from build123d import *

# Parameters (mm, degrees)
F1_DEPTH  = 31.6
F2_START  = 27.6
F2_DEPTH  = 4
F0_R      = 3.05
F3_DEPTH  = 2
F4_W      = 2.5
F4_H      = 19.6
F5_DEPTH  = 2
F7_DEPTH  = 3
F8_R      = 0.5
F9_DEPTH  = 25
F10_R     = 1.75
F11_DEPTH = 3
F13_DEPTH = 10
F15_DEPTH = 4


# Not quite as in the source:
# - a feature names something its author has since deleted; it is built from what else it names


with BuildPart() as f1:
    # F0 (on Top) → F1 (new body)
    with BuildSketch(Plane.XY):
        Polygon((31.25, -9), (31.25, 0), (29.25, 0), (29.25, -7), (-29.25, -7), (-29.25, 0), (-31.25, 0), (-31.25, -9), align=None)
        Polygon((31.25, 0), (31.25, 9), (-31.25, 9), (-31.25, 0), (-29.25, 0), (-29.25, 7), (29.25, 7), (29.25, 0), align=None)
    extrude(amount=F1_DEPTH)

    # F0 (on Top) → F2 (join)
    with BuildSketch(Plane.XY.offset(F2_START)):
        with BuildLine():
            Line((29, 0), (29.25, 0))
            Line((29.25, 0), (29.25, 7))
            Line((29.25, 7), (-29.25, 7))
            Line((-29.25, 7), (-29.25, 0))
            Line((-29.25, 0), (-29, 0))
            ThreePointArc((-29, 0), (-24.5, 4.5), (-20, 0))
            Line((-20, 0), (-16.1, 0))
            ThreePointArc((-16.1, 0), (-13.5, 2.6), (-10.9, 0))
            Line((-10.9, 0), (-7.1, 0))
            ThreePointArc((-7.1, 0), (-4.5, 2.6), (-1.9, 0))
            Line((-1.9, 0), (0, 0))
            Line((0, 0), (1.9, 0))
            ThreePointArc((1.9, 0), (4.5, 2.6), (7.1, 0))
            Line((7.1, 0), (10.9, 0))
            ThreePointArc((10.9, 0), (13.5, 2.6), (16.1, 0))
            Line((16.1, 0), (20, 0))
            ThreePointArc((20, 0), (24.5, 4.5), (29, 0))
        make_face()
        with BuildLine():
            Line((29.25, -7), (29.25, 0))
            Line((29.25, 0), (29, 0))
            ThreePointArc((29, 0), (24.5, -4.5), (20, 0))
            Line((20, 0), (16.1, 0))
            ThreePointArc((16.1, 0), (13.5, -2.6), (10.9, 0))
            Line((10.9, 0), (7.1, 0))
            ThreePointArc((7.1, 0), (4.5, -2.6), (1.9, 0))
            Line((1.9, 0), (0, 0))
            Line((0, 0), (-1.9, 0))
            ThreePointArc((-1.9, 0), (-4.5, -2.6), (-7.1, 0))
            Line((-7.1, 0), (-10.9, 0))
            ThreePointArc((-10.9, 0), (-13.5, -2.6), (-16.1, 0))
            Line((-16.1, 0), (-20, 0))
            ThreePointArc((-20, 0), (-24.5, -4.5), (-29, 0))
            Line((-29, 0), (-29.25, 0))
            Line((-29.25, 0), (-29.25, -7))
            Line((-29.25, -7), (29.25, -7))
        make_face()
    extrude(amount=F2_DEPTH)

    # F0 (on Top) → F3 (join)
    with BuildSketch(Plane.XY):
        Polygon((-41.25, 19), (-41.25, 14), (-41.25, -19), (41.25, -19), (41.25, 19), align=None)
        with Locations((-27.5, 14)):
            Circle(F0_R, mode=Mode.SUBTRACT)
        Polygon((-31.25, 9), (31.25, 9), (31.25, 0), (31.25, -9), (-31.25, -9), (-31.25, 0), align=None, mode=Mode.SUBTRACT)
        with Locations((27.5, 14)):
            Circle(F0_R, mode=Mode.SUBTRACT)
    extrude(amount=F3_DEPTH)

    # F4 (on face) → F5 (cut)
    with BuildSketch(Plane.XZ.offset(9)):
        with Locations((-1.25, 21.8)):
            Rectangle(F4_W, F4_H)
        with Locations((1.25, 21.8)):
            Rectangle(F4_W, F4_H)
    extrude(amount=-F5_DEPTH, mode=Mode.SUBTRACT)

    # F6 (on face) → F7 (join)
    with BuildSketch(Plane.XY.offset(31.6)):
        Polygon((-27, -6), (-27, -9), (-25, -9), (-23, -9), (-23, -6), (-25, -6), align=None)
        Polygon((23, -6), (23, -9), (25, -9), (27, -9), (27, -6), (25, -6), align=None)
        Polygon((-23, 6), (-23, 9), (-25, 9), (-27, 9), (-27, 6), (-25, 6), align=None)
        Polygon((25, 6), (27, 6), (27, 9), (25, 9), (23, 9), (23, 6), align=None)
    extrude(amount=F7_DEPTH)

    # F8 (on face) → F9 (cut)
    with BuildSketch(Plane.XZ.offset(9)):
        with BuildLine():
            ThreePointArc((-25, 33.6), (-25.3535533906, 32.7464466094), (-24.5, 33.1))
            ThreePointArc((-24.5, 33.1), (-24.6464466094, 33.4535533906), (-25, 33.6))
        make_face()
        with Locations((25, 33.1)):
            Circle(F8_R)
    extrude(amount=-F9_DEPTH, mode=Mode.SUBTRACT)

    # F10 (on face) → F11 (join)
    with BuildSketch(Plane.YZ.offset(31.25)):
        with Locations((5, 8)):
            Circle(F10_R)
    extrude(amount=F11_DEPTH)

    # F12 (on face) → F13 (join)
    with BuildSketch(Plane.XY.offset(2)):
        Polygon((-11.5, -9), (-15.5, -9), (-15.5, -11), (-15.5, -14), (0, -14), (15.5, -14), (15.5, -11), (15.5, -9), (11.5, -9), (11.5, -12), (0, -12), (-11.5, -12), align=None)
    extrude(amount=F13_DEPTH)

    # F14 (on face) → F15 (cut)
    with BuildSketch(Plane.XZ.offset(14)):
        Polygon((-10, 2), (0, 2), (10, 2), (10, 8), (0, 8), (-10, 8), align=None)
    extrude(amount=-F15_DEPTH, mode=Mode.SUBTRACT)


solid = f1.part
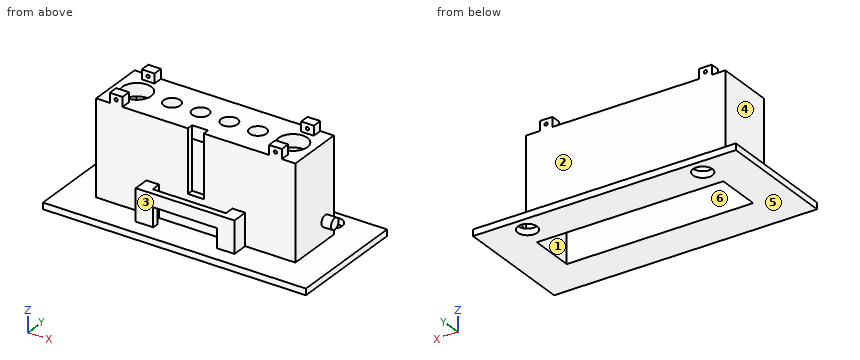
The listing builds one solid part. Answer for the finished solid, in the listing's coordinates (mm). Face numbers are marked on the shaded views. A direction names the side the tool comes from. Coordinates: 2 decimals unless noted, no trailing zeros. Order: outer loops, then holes, each group sorted by start corner. A loop starts at its lowest first (then second) coordinate and runs counter-clockwise, first axis right, second up.
Q1. A cutting plane is placed at C-C, the plane x = -4.5. Write down the section's boundary in (y, z).
Q2. Consider line 1 (X direction, y = -7.6, z = 33.1); line 2 (Y direction, x = 4.5, z = 30.8); line 3 (Y direction, x = -16.5, z = 10.5). Determine where each line is inside the solid, lowest interval first.
Q3. For a pull along Y with two mould halves and no side action, classify the marked faces 1, 2, 3 and 4 as pulls with the +Y half, pulls with the -Y half, needs draft (parallel to the pull), parting line crosses it, or undercut.
Q4. A cutting plane is placed at B-B, the plane z = 29. Write down the section's boundary in (x, y).
Q5. A cutting plane is placed at D-D, the plane y = 15. Write down the section's boundary in (x, z).
Q6. Which of the six approach directions +Z, -Z, +X, -X, +Y, -Y give full straight-line access (tool end or side, diameter ignored) to the marked faces 5 and 6?
Q7. A cutting plane is placed at A-A, the plane x = -13.5. Write down the section's boundary in (y, z).
Q8. Given P1, Ø4, axis at x = 11.5, z = 26, coming from the -Y side; P2, Ø2, axis at x = -23, y = -3.5, coming from the +Z side; P3, Ø0.6, axis at y = -8, z = 24.5, coming from the -X side; P4, Ø2, axis at x = -0.5, y = -12.5, coming from the -Z side, each flat-ended and moving along its own axis, determine where each tip first touches the part or whether it passes through.
Answers follow:
1. outline: (-19, 0) - (-7, 0) - (-7, 27.6) - (-2.6, 27.6) - (-2.6, 31.6) - (-9, 31.6) - (-9, 2) - (-19, 2) - close; (-14, 8) - (-12, 8) - (-12, 12) - (-14, 12) - close; (2.6, 27.6) - (7, 27.6) - (7, 0) - (19, 0) - (19, 2) - (9, 2) - (9, 31.6) - (2.6, 31.6) - close
2. line 1: x = -27 to -25.5, -24.5 to -23, 23 to 24.5, 25.5 to 27
2. line 2: y = -9 to -2.6, 2.6 to 9
2. line 3: y = -9 to -7, 7 to 9
3. face 1: undercut
3. face 2: pulls with the +Y half
3. face 3: pulls with the -Y half
3. face 4: needs draft
4. outline: (-31.25, -9) - (-2.5, -9) - (-2.5, -7) - (2.5, -7) - (2.5, -9) - (31.25, -9) - (31.25, 9) - (-31.25, 9) - close; hole circle Ø9 at (-24.5, 0); hole circle Ø5.2 at (-13.5, 0); hole circle Ø5.2 at (-4.5, 0); hole circle Ø5.2 at (4.5, 0); hole circle Ø5.2 at (13.5, 0); hole circle Ø9 at (24.5, 0)
5. outline: (-41.25, 0) - (-30.38, 0) - (-30.38, 2) - (-41.25, 2) - close; (-24.62, 0) - (24.62, 0) - (24.62, 2) - (-24.62, 2) - close; (30.38, 0) - (41.25, 0) - (41.25, 2) - (30.38, 2) - close
6. face 5: -Z, +X, -X, +Y, -Y
6. face 6: -Z
7. outline: (-19, 0) - (-7, 0) - (-7, 27.6) - (-2.6, 27.6) - (-2.6, 31.6) - (-9, 31.6) - (-9, 12) - (-14, 12) - (-14, 2) - (-19, 2) - close; (2.6, 27.6) - (7, 27.6) - (7, 0) - (19, 0) - (19, 2) - (9, 2) - (9, 31.6) - (2.6, 31.6) - close
8. P1: stops at y = -9
8. P2: stops at z = 31.6
8. P3: stops at x = -31.25
8. P4: stops at z = 0
